```python
from build123d import *

# Parameters (mm, degrees)
F0_R     = 12.7
F1_DEPTH = 12.7


with BuildPart() as f1:
    # F0 (on Top) → F1 (new body)
    with BuildSketch(Plane.XY):
        with BuildLine():
            Line((-6.35, 25.4), (-6.35, 37.567107))
            ThreePointArc((-6.35, 37.567107), (-32.995568, 19.05), (-35.709069, -13.284292))
            Line((-35.709069, -13.284292), (-25.172045, -7.200739))
            Line((-25.172045, -7.200739), (-18.822045, -18.199261))
            Line((-18.822045, -18.199261), (-29.359069, -24.282815))
            ThreePointArc((-29.359069, -24.282815), (0, -38.1), (29.359069, -24.282815))
            Line((29.359069, -24.282815), (18.822045, -18.199261))
            Line((18.822045, -18.199261), (25.172045, -7.200739))
            Line((25.172045, -7.200739), (35.709069, -13.284292))
            ThreePointArc((35.709069, -13.284292), (32.995568, 19.05), (6.35, 37.567107))
            Line((6.35, 37.567107), (6.35, 25.4))
            Line((6.35, 25.4), (-6.35, 25.4))
        make_face()
        Circle(F0_R, mode=Mode.SUBTRACT)
    extrude(amount=F1_DEPTH)


solid = f1.part
```
Geometry: final body of the model. Coordinates: model frame, mm. A direction names the side the tool comes from. Give positions to 0.01 mm unless a question says otherwise; leave off trailing zeros. Write each loop counter-clockwise with the first axis right and the second up, starting at its lowest first coordinate (ties: lowest second). Pieces come first, ordered by that corner, then holes.
1. Pin query (flat end, axial travel): P1, Ø1.5, axis at y = 14, z = 8, coming from the -X side; P2, Ø6, axis at y = 25.5, z = 5.5, coming from the -X side; P3, Ø10, axis at x = 30, y = -17, coming from the +Z side; P4, Ø6, axis at x = -4, z = 5.5, coming from the +Y side. Return the tip coordinate at first contact, or that it passes through.
2. Line query: probe 1 along Y at (x, z) = (0, 6.75); probe 2 along X at (y, z) = (-8, 7.5); probe 3 along Y at (x, z) = (-2.5, 1.75). Output: solid intervals per line, ascending.
3. Section query A-A, the plane x = 0. Return loops of the section in (y, z).
4. Section query D-D, the plane y = -31.5. Return loops of the section in (x, z).
5. Reachability of faces 1 (the cylindrical face through (-0.469, -38.097, 6.261)), 2 (the flat face through (-6.35, 31, 6)), 3 (the flat face through (30.37, -10.2, 6.26)), 4 (the flat face through (-24.02, -21.2, 6.26)), 5 (the cylindrical face through (33.23, 18.64, 6.26)) from +Z, -Z, +X, -X, +Y, -Y: full face, straight path, thin tool, end or side. Return the list, or none.
6. Draft query along X for faces 6 (the cylindrical face through (-32.76, 19.45, 6.26)), 7 (the cylindrical face through (-2.75, -12.4, 6.26)), 8 (the flat face through (24.16, -21.28, 6.26)), 9 (the flat face through (21.95, -12.78, 6.26)). Return one class per face: released by +X, released by -X, zero draft, split by the parting line, or undercut.
7. Section query C-C, the plane z = 10. Return loops of the section in (x, y), then the cut area to 3 significant figures.
8. Section query B-B, the plane y = 0. Return loops of the section in (x, z), then the cut area to 3 significant figures.
Computed:
1. P1: stops at x = -35.72
1. P2: stops at x = -30.75
1. P3: passes through
1. P4: stops at y = 37.57
2. probe 1: y = -38.1 to -12.7, 12.7 to 25.4
2. probe 2: x = -37.25 to -26.56, -24.71 to -9.86, 9.86 to 24.71, 26.56 to 37.25
2. probe 3: y = -38.02 to -12.45, 12.45 to 25.4
3. outline: (-38.1, 0) - (-12.7, 0) - (-12.7, 12.7) - (-38.1, 12.7) - close; (12.7, 0) - (25.4, 0) - (25.4, 12.7) - (12.7, 12.7) - close
4. outline: (-21.43, 0) - (21.43, 0) - (21.43, 12.7) - (-21.43, 12.7) - close
5. face 1: +Z, -Z, -Y
5. face 2: +Z, -Z, +Y
5. face 3: +Z, -Z
5. face 4: +Z, -Z, -X
5. face 5: +Z, -Z, +X
6. face 6: released by -X
6. face 7: undercut
6. face 8: released by +X
6. face 9: undercut
7. outline: (-35.71, -13.28) - (-25.17, -7.2) - (-18.82, -18.2) - (-29.36, -24.28) arc R38.1 ccw to (29.36, -24.28) - (18.82, -18.2) - (25.17, -7.2) - (35.71, -13.28) arc R38.1 ccw to (6.35, 37.57) - (6.35, 25.4) - (-6.35, 25.4) - (-6.35, 37.57) arc R38.1 ccw to start; hole circle Ø25.4 at (0, 0)
7. area: 3,580 mm2
8. outline: (-38.1, 0) - (-12.7, 0) - (-12.7, 12.7) - (-38.1, 12.7) - close; (12.7, 0) - (38.1, 0) - (38.1, 12.7) - (12.7, 12.7) - close
8. area: 645 mm2
